```python
from build123d import *

# Parameters (mm, degrees)
BASE_VOLUME_DEPTH   = 10
WEIGHT_SAVING_REACH = 140.59
D_SHAFT_HOLE_REACH  = 140.062
TROUS_M3_DEPTH      = 139.273289153
TROUS_M3_DEPTH_BACK = 139.273289153
SKETCH15_R          = 1.5


with BuildPart() as part:
    # Sketch9 → base_volume (new body)
    with BuildSketch(Plane.XY):
        with BuildLine():
            Line((-2.24506403, 2.24506403), (2.24506403, -2.24506403))
            Line((2.24506403, -2.24506403), (86.830152477, 82.340024416))
            ThreePointArc((86.830152477, 82.340024416), (86.087387236, 100.986393717), (67.559180599, 98.762804922))
            Line((67.559180599, 98.762804922), (-2.24506403, 2.24506403))
        make_face()
    base_volume = extrude(amount=-BASE_VOLUME_DEPTH)

    # weight_saving: up to this plane
    weight_saving_end = Plane(origin=(2.24506403, -2.24506403, -10), z_dir=(0.7071067811865464, -0.7071067811865487, 0))
    # Sketch10 → weight_saving (cut, up to the surface)
    with BuildSketch(Plane(origin=(-2.540124292, 1.837086693, 0), x_dir=(0, 0, 1), z_dir=(-0.8102925792823216, 0.5860255420713356, 0)), mode=Mode.PRIVATE) as weight_saving_sk1:
        Polygon((-5, -0.503493858), (-10, 107.3), (-10, -0.503493858), align=None)
    weight_saving_tool1 = split(extrude(weight_saving_sk1.sketch, amount=-WEIGHT_SAVING_REACH, mode=Mode.PRIVATE), bisect_by=weight_saving_end, keep=Keep.BOTH, mode=Mode.PRIVATE)
    # Sketch10 → weight_saving (cut, up to the surface)
    with BuildSketch(Plane(origin=(-2.540124292, 1.837086693, 0), x_dir=(0, 0, 1), z_dir=(-0.8102925792823216, 0.5860255420713356, 0)), mode=Mode.PRIVATE) as weight_saving_sk2:
        Polygon((0, 83), (0, 132.318173369), (-6.45, 132.318173369), (-6.45, 92.318173369), (-5.949148181, 83), align=None)
    weight_saving_tool2 = split(extrude(weight_saving_sk2.sketch, amount=-WEIGHT_SAVING_REACH, mode=Mode.PRIVATE), bisect_by=weight_saving_end, keep=Keep.BOTH, mode=Mode.PRIVATE)
    # Sketch10 → weight_saving (cut, up to the surface)
    with BuildSketch(Plane(origin=(-2.540124292, 1.837086693, 0), x_dir=(0, 0, 1), z_dir=(-0.8102925792823216, 0.5860255420713356, 0)), mode=Mode.PRIVATE) as weight_saving_sk3:
        Polygon((0, 32.318173369), (0, 77), (-5.626648181, 77), (-3.225, 32.318173369), align=None)
    weight_saving_tool3 = split(extrude(weight_saving_sk3.sketch, amount=-WEIGHT_SAVING_REACH, mode=Mode.PRIVATE), bisect_by=weight_saving_end, keep=Keep.BOTH, mode=Mode.PRIVATE)
    weight_saving = weight_saving_tool1.solids().sort_by_distance((18.223349, 30.546566, -8.333333))[0] + weight_saving_tool2.solids().sort_by_distance((60.64419, 89.201506, -3.202401))[0] + weight_saving_tool3.solids().sort_by_distance((30.675578, 47.764158, -2.267214))[0]
    add(weight_saving, mode=Mode.SUBTRACT)

    # Sketch11 → D-shaft_hole (cut, up to next)
    with BuildSketch(Plane.XY.offset(-6.45), mode=Mode.PRIVATE) as d_shaft_hole_sk1:
        with BuildLine():
            Line((75.954896356, 93.86774987), (79.744896356, 93.86774987))
            ThreePointArc((79.744896356, 93.86774987), (77.849896356, 88.145280537), (75.954896356, 93.86774987))
        make_face()
    d_shaft_hole_tool1 = extrude(d_shaft_hole_sk1.sketch, amount=-D_SHAFT_HOLE_REACH, mode=Mode.PRIVATE) & part.part
    d_shaft_hole = d_shaft_hole_tool1.solids().sort_by_distance((77.849896, 91.169307, -6.45))[0]
    add(d_shaft_hole, mode=Mode.SUBTRACT)

    # Mirror1: base_volume, weight_saving, D-shaft_hole across plane
    add(base_volume.mirror(Plane.XY))
    add(weight_saving.mirror(Plane.XY), mode=Mode.SUBTRACT)
    add(d_shaft_hole.mirror(Plane.XY), mode=Mode.SUBTRACT)

    # Sketch15 → trous_m3 (cut, two sides: drawn at the far end of the back side and taken through both)
    with BuildSketch(Plane.XY.offset(-TROUS_M3_DEPTH_BACK)):
        with Locations(Location((5.268760152, 6.160633141, 0), (0, 0, 54.124527059))):
            Circle(SKETCH15_R)
        with Locations(Location((15.806280456, 18.481899424, 0), (0, 0, 54.124527059))):
            Circle(SKETCH15_R)
        with Locations(Location((49.527674377, 62.910014332, 0), (0, 0, 54.124527059))):
            Circle(SKETCH15_R)
        with Locations(Location((54.713429681, 59.159535628, 0), (0, 0, 54.124527059))):
            Circle(SKETCH15_R)
    extrude(amount=TROUS_M3_DEPTH + TROUS_M3_DEPTH_BACK, mode=Mode.SUBTRACT)


solid = part.part
```
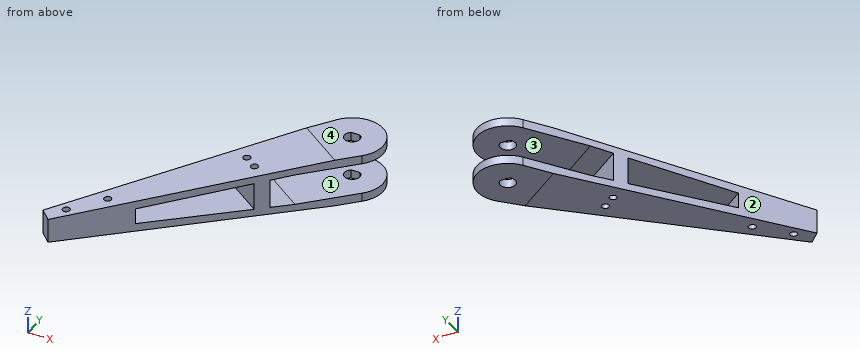
Geometry check sheet. Reference: the model listing, model coordinates, mm. Face numbers are marked on the shaded views. Coordinates: 2 decimals unless noted, no trailing zeros. Order: outer loops, then holes, each group sorted by start corner. A loop starts at its lowest first (then second) coordinate and runs counter-clockwise, first axis right, second up. Notation, with made-up numbers: (-2, 5) - (36, 5) arc R38 ccw to (36, 43) - close; hole circle Ø6 at (-18.75, -13). An arc over 180 degrees is marked (long way). Answer as a JSON object with one key per item and string values. Group by question number.
Item 1: Depth check by flat-ended pin: pin 1 Ø1.1 at (x, z) = (77.5, -8.5) entering from -Y; pin 2 Ø5 at (x, z) = (21.5, 6.5) entering from +Y; pin 3 Ø1.8 at (x, y) = (54.71, 59.16) entering from +Z; pin 4 Ø3 at (x, z) = (66.5, -5.5) entering from +Y. Enter the tip coordinate at first touch or a pass-through.
Item 2: Sectioned sample at B-B, the plane y = 72.5. Record the cut outline in (x, z), and give its area (3 significant figures).
Item 3: Sectioned sample at A-A, the plane x = 30. Record the cut outline in (y, z), and give its area (3 significant figures).
Item 4: Sectioned sample at C-C, the plane x = 70. Record the cut outline in (y, z), and give its area (3 significant figures).
Item 5: Sectioned sample at D-D, the plane y = 43. Record the cut outline in (x, z).
Item 6: Scan lines: probe 1 along Z at (x, y) = (51, 53); probe 2 along Z at (x, y) = (48.5, 50.5); probe 3 along Y at (x, z) = (4.5, 2). Record each from-to range of solid material in increasing order.
Item 7: Draft check along Z on the marked faces 1, 2, 3 and 4. Enter one of: +Z half, -Z half, draft (parallel to the pull), parting line (faces both ways), or undercut.
Resolved:
{
 "1": {"pin 1": "y = 72.46", "pin 2": "y = 38.53", "pin 3": "through", "pin 4": "y = 98.9"},
 "2": {"outline": "(48.57, -9.07) - (76.99, -9.84) - (76.99, -6.45) - (57.29, -6.45) - (48.57, -6.18) - close; (48.57, 6.18) - (57.29, 6.45) - (76.99, 6.45) - (76.99, 9.84) - (48.57, 9.07) - close", "area": "173 mm^2"},
 "3": {"outline": "(25.51, -6.8) - (46.83, -7.6) - (46.83, -4.47) - (25.51, -3.54) - close; (25.51, 3.54) - (46.83, 4.47) - (46.83, 7.6) - (25.51, 6.8) - close", "area": "136 mm^2"},
 "4": {"outline": "(65.51, -9.39) - (81.8, -10) - (101.3, -10) - (101.3, -6.45) - (65.51, -6.45) - close; (65.51, 6.45) - (101.3, 6.45) - (101.3, 10) - (81.8, 10) - (65.51, 9.39) - close", "area": "244 mm^2"},
 "5": {"outline": "(27.23, -7.38) - (47.49, -7.93) - (47.49, -4.86) - (27.23, -4.22) - close; (27.23, 4.22) - (47.49, 4.86) - (47.49, 7.93) - (27.23, 7.38) - close"},
 "6": {"probe 1": "-8.4 to -5.4, 5.4 to 8.4", "probe 2": "-8.24 to -5.22, 5.22 to 8.24", "probe 3": "0.01 to 4.87, 7.45 to 11.57"},
 "7": {"face 1": "undercut", "face 2": "draft", "face 3": "undercut", "face 4": "+Z half"}
}
